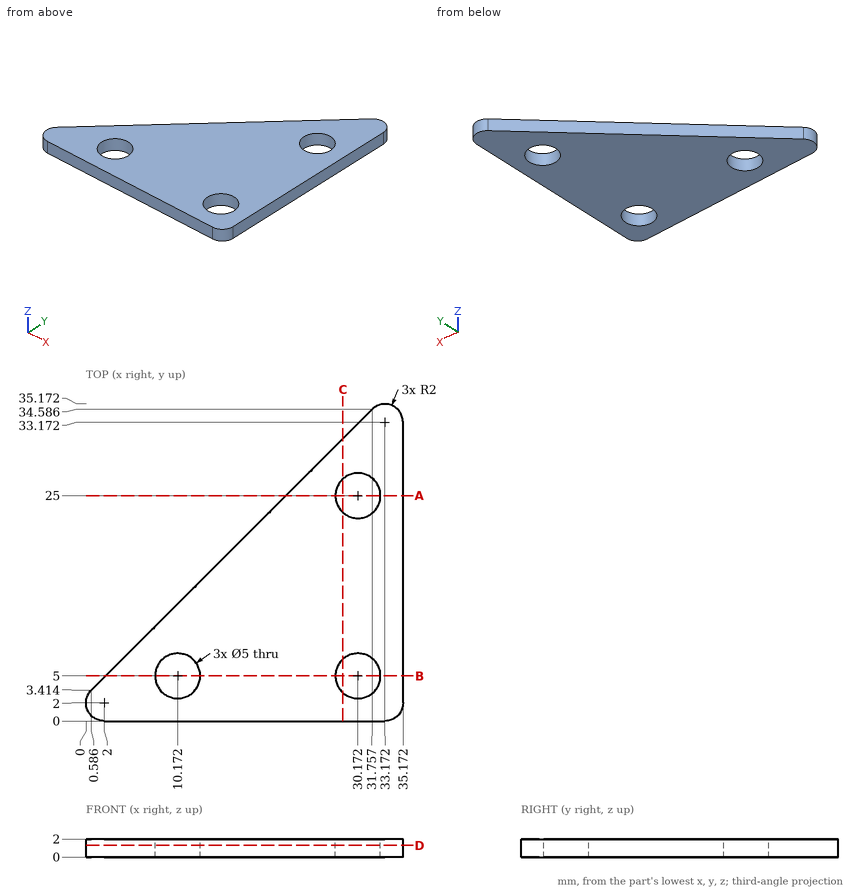
Geometry: see drawing. Coordinates: mm, zero at the bounding-box minimum. Coordinates: 2 decimals unless noted, no trailing zeros. Loops run counter-clockwise (first coordinate to the right, second up) from the corner with the lowest first, then second, coordinate; pieces in that order, holes last. Notation, with made-up numbers: (20, 23) - (44, 23) arc R34 cw to (44, 62) - close; hole circle Ø10 at (-15, 51.5). An arc over 180 degrees is marked (long way). Answer as CSV lines item,"result".
1. Section D-D (z = 1.3). Return loops of the section in (x, y) (1 decimal), then the cut area to 3 significant figures.
Established:
outline,"(0.6, 3.4) arc R2 ccw to (2, 0) - (33.2, 0) arc R2 ccw to (35.2, 2) - (35.2, 33.2) arc R2 ccw to (31.8, 34.6) - close; hole circle Ø5 at (10.2, 5); hole circle Ø5 at (30.2, 5); hole circle Ø5 at (30.2, 25)"
area,"652 mm2"
2. Section B-B (y = 5). Return loops of the section in (x, z).
Established:
outline,"(2.17, 0) - (7.67, 0) - (7.67, 2) - (2.17, 2) - close; (12.67, 0) - (27.67, 0) - (27.67, 2) - (12.67, 2) - close; (32.67, 0) - (35.17, 0) - (35.17, 2) - (32.67, 2) - close"
3. Section C-C (x = 28.5). Return loops of the section in (y, z).
Established:
outline,"(0, 0) - (3.14, 0) - (3.14, 2) - (0, 2) - close; (6.86, 0) - (23.14, 0) - (23.14, 2) - (6.86, 2) - close; (26.86, 0) - (31.33, 0) - (31.33, 2) - (26.86, 2) - close"
4. Section A-A (y = 25). Return loops of the section in (x, z).
Established:
outline,"(22.17, 0) - (27.67, 0) - (27.67, 2) - (22.17, 2) - close; (32.67, 0) - (35.17, 0) - (35.17, 2) - (32.67, 2) - close"
5. Contact query for flat-ended pins moving along their axis: pin 1 (8 mm diameter, centred on x = 25.5, y = 8, fed in from -Z); pin 2 (1 mm diameter, centred on y = 9.5, z = 1, fed in from -X). Output: stop coordinate, or through.
Established:
pin 1,"stops at z = 0"
pin 2,"stops at x = 6.17"
6. Ray query, line 1 (X direction, y = 3, z = 1) (1 decimal); line 2 (Y direction, x = 28, z = 0.15) (1 decimal); line 3 (X direction, y = 25.5, z = 1.85). Return the intervals inside material, ascending.
Established:
line 1,"x = 0.3 to 8.7, 11.7 to 28.7, 31.7 to 35.2"
line 2,"y = 0 to 3.8, 6.2 to 23.8, 26.2 to 30.8"
line 3,"x = 22.67 to 27.72, 32.62 to 35.17"
